from build123d import *

# Parameters (mm, degrees)
SKETCH1_R           = 6.5
SKETCH1_R_2         = 3.5
BOSS_EXTRUDE1_DEPTH = 7
SKETCH2_R           = 9.5
SKETCH2_R_2         = 3.503174071
BOSS_EXTRUDE3_DEPTH = 4
CHAMFER1_SIZE       = 0.5
FILLET1_R           = 0.5


with BuildPart() as part:
    # Sketch1 → Boss-Extrude1 (new body)
    with BuildSketch(Plane(origin=(0, 0, 0), x_dir=(1, 0, 0), z_dir=(0, 1, 0))):
        with Locations(Location((0, 0, 0), (0, 0, 270))):
            Circle(SKETCH1_R)
        with Locations(Location((0, 0, 0), (0, 0, 270))):
            Circle(SKETCH1_R_2, mode=Mode.SUBTRACT)
    extrude(amount=BOSS_EXTRUDE1_DEPTH)

    # Sketch2 → Boss-Extrude3 (add)
    with BuildSketch(Plane(origin=(0, 7, 0), x_dir=(1, 0, 0), z_dir=(0, 1, 0))):
        with Locations(Location((0, 0, 0), (0, 0, 270))):
            Circle(SKETCH2_R)
        with Locations(Location((0, 0, 0), (0, 0, 270))):
            Circle(SKETCH2_R_2, mode=Mode.SUBTRACT)
    extrude(amount=BOSS_EXTRUDE3_DEPTH)

    # Chamfer1
    chamfer1_edges = [part.edges().sort_by_distance(p)[0] for p in [
        (0, 11, -3.503174071),
    ]]
    chamfer(chamfer1_edges, length=CHAMFER1_SIZE)

    # Fillet1
    fillet1_edges = [part.edges().sort_by_distance(p)[0] for p in [
        (0, 11, -9.5),
    ]]
    fillet(fillet1_edges, radius=FILLET1_R)


solid = part.part
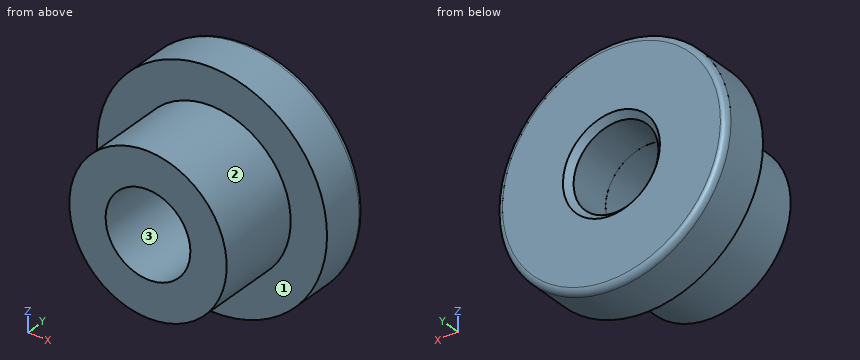
Geometry check sheet. Reference: the model listing, model coordinates, mm. Face numbers are marked on the shaded views. Give positions to 0.01 mm unless a question says otherwise; leave off trailing zeros. Order: outer loops, then holes, each group sorted by start corner. A loop starts at its lowest first (then second) coordinate and runs counter-clockwise, first axis right, second up.
1. Depth check by flat-ended pin: pin 1 (3 mm diameter, centred on y = 5, z = -7.5, fed in from -X); pin 2 (4 mm diameter, centred on x = 5, y = 3.5, fed in from -Z); pin 3 (2 mm diameter, centred on y = 1.5, z = -1, fed in from +X). Enter the tip coordinate at first touch or a pass-through.
Completed:
pin 1: stops at x = -2.5
pin 2: stops at z = -5.77
pin 3: stops at x = 6.5
2. Sectioned sample at D-D (y = 5). Record the boundary of the cut face in (x, z).
Completed:
outline: circle Ø13 at (0, 0); hole circle Ø7 at (0, 0)
3. Sectioned sample at C-C (y = 8.75). Record the boundary of the cut face in (x, z), then the cut area to 3 significant figures.
Completed:
outline: circle Ø19 at (0, 0); hole circle Ø7.01 at (0, 0)
area: 245 mm2
4. Scan lines: line 1 (X direction, y = 2.25, z = 0); line 2 (X direction, y = 8.45, z = 0); line 3 (Y direction, x = -7.25, z = -2.5). Record each from-to range of solid material in increasing order.
Completed:
line 1: x = -6.5 to -3.5, 3.5 to 6.5
line 2: x = -9.5 to -3.5, 3.5 to 9.5
line 3: y = 7 to 11
5. Draft check along X on the marked faces 1, 2 and 3. Enter one of: pulls with the +X half, pulls with the -X half, needs draft (parallel to the pull), parting line crosses it, or undercut.
Completed:
face 1: needs draft
face 2: parting line crosses it
face 3: undercut
